from build123d import *

# Parameters (mm, degrees)
EXTRUDE_1_DEPTH     = 2
CUT_EXTRUDE_2_DEPTH = 3


with BuildPart() as part:
    # Эскиз2 → Бобышка-Вытянуть1 (new body)
    with BuildSketch(Plane(origin=(0, 0, 0), x_dir=(1, 0, 0), z_dir=(0, 1, 0))):
        with BuildLine():
            ThreePointArc((-34.560822595, -73.294650793), (-29.912438938, -99.847233064), (-35.042219755, -126.311028042))
            ThreePointArc((-35.042219755, -126.311028042), (-8.723554926, -145.4763519), (4.999999999, -175))
            ThreePointArc((4.999999999, -175), (18.723554924, -145.4763519), (45.042219753, -126.311028042))
            ThreePointArc((45.042219753, -126.311028042), (39.912438936, -99.847233064), (44.560822593, -73.294650793))
            ThreePointArc((44.560822593, -73.294650793), (19.227048475, -55.497690672), (4.999999999, -28))
            ThreePointArc((4.999999999, -28), (-9.227048477, -55.497690672), (-34.560822595, -73.294650793))
        make_face()
    extrude(amount=EXTRUDE_1_DEPTH)

    # Эскиз5 → Вырез-Вытянуть2 (cut, through all)
    with BuildSketch(Plane(origin=(0, 2, 0), x_dir=(1, 0, 0), z_dir=(0, 1, 0))):
        with BuildLine():
            ThreePointArc((1.1922114, -102.391848867), (9.263771174, -100.007354542), (1.1922114, -97.622860217))
            ThreePointArc((1.1922114, -97.622860217), (3.802790428, -100.007354542), (1.1922114, -102.391848867))
        make_face()
        with BuildLine():
            ThreePointArc((-1.894766012, -94.327614743), (4.875778497, -91.169950109), (11.646323005, -94.327614743))
            add(Edge.make_bspline(
                [(11.646323005, -94.327614743), (10.113303771, -87.718633088), (4.875778497, -83.368495621)],
                knots=[0, 0, 0, 1, 1, 1], degree=2))
            add(Edge.make_bspline(
                [(-1.894766012, -94.327614743), (-0.361746778, -87.718633088), (4.875778497, -83.368495621)],
                knots=[0, 0, 0, 1, 1, 1], degree=2))
        make_face()
        with BuildLine():
            add(Edge.make_bspline(
                [(11.646323005, -105.687094341), (10.113303771, -112.296075996), (4.875778497, -116.646213463)],
                knots=[0, 0, 0, 1, 1, 1], degree=2))
            ThreePointArc((11.646323005, -105.687094341), (4.875778497, -108.844758976), (-1.894766012, -105.687094341))
            add(Edge.make_bspline(
                [(-1.894766012, -105.687094341), (-0.361746778, -112.296075996), (4.875778497, -116.646213463)],
                knots=[0, 0, 0, 1, 1, 1], degree=2))
        make_face()
        with BuildLine():
            ThreePointArc((6.916781621, -81.95103194), (14.912317424, -99.810070996), (7.206797889, -117.796144427))
            add(Edge.make_bspline(
                [(6.916781621, -81.95103194), (12.307611516, -78.787526654), (22.389316178, -80.793310488), (29.731357531, -92.811077081), (30.434704422, -105.116682284), (25.64381117, -115.001664232), (17.091486552, -120.227210357), (10.646188457, -120.056173748), (7.206797889, -117.796144427)],
                knots=[0, 0, 0, 0, 0.238043411, 0.386081267, 0.575651621, 0.751375083, 0.825495316, 1, 1, 1, 1], degree=3))
        make_face()
        with BuildLine():
            ThreePointArc((2.544759104, -117.796144427), (-5.160760431, -99.810070996), (2.834775372, -81.95103194))
            add(Edge.make_bspline(
                [(2.834775372, -81.95103194), (-2.556054523, -78.787526654), (-12.637759184, -80.793310488), (-19.979800538, -92.811077081), (-20.683147428, -105.116682284), (-15.892254177, -115.001664232), (-7.339929559, -120.227210357), (-0.894631464, -120.056173748), (2.544759104, -117.796144427)],
                knots=[0, 0, 0, 0, 0.238043411, 0.386081267, 0.575651621, 0.751375083, 0.825495316, 1, 1, 1, 1], degree=3))
        make_face()
    extrude(amount=-CUT_EXTRUDE_2_DEPTH, mode=Mode.SUBTRACT)


solid = part.part
Part model, mm, in its own coordinate system. Coordinates: 2 decimals unless noted, no trailing zeros. Order: outer loops, then holes, each group sorted by start corner. A loop starts at its lowest first (then second) coordinate and runs counter-clockwise, first axis right, second up. Notation, with made-up numbers: M 50.5,76.5 L 84.5,76.5 A12 ccw 84.5,87.5 Z; hole C -2.5,55 d5. An arc over 180 degrees is marked long. One line per question, with ' | ' between items.
Q1. Two-plate mould, pull along X, no slides. Class faces 1 (the face through (9.26, 1.01, 100.17)), 2 (the face through (19.52, 0.99, 55.83)), 3 (the face through (-8.94, 0.986, 55.167)): +X half, -X half, draft (parallel to the pull), parting line (faces both ways), or undercut.
A:
face 1: undercut | face 2: +X half | face 3: -X half
Q2. Drill centre lines: line 1 (X direction, y = 1.9, z = 95); line 2 (Z direction, x = -0.5, y = 1.6); line 3 (X direction, y = 0.4, z = 91). Where is each one in solid material? Low to high.
A:
line 1: x = -30.03 to -19.51, -4.64 to 14.39, 29.26 to 40.03 | line 2: z = 42.7 to 80.56, 85.67 to 90.26, 92.99 to 107.02, 109.76 to 114.35, 119.19 to 158.28 | line 3: x = -30.36 to -18.28, -3.44 to -0.83, 10.58 to 13.19, 28.03 to 40.36
Q3. Slice it at C-C (z = 41). Give the cut face in (x, y).
A:
outline: M 0.35,0 L 9.65,0 L 9.65,2 L 0.35,2 Z
Q4. Slice it at A-A (z = 88). Count the separate pieces of the cut face and the enclosed holes in it, and give its area (3 significant figures).
A:
separate pieces: 4 | enclosed holes: 0 | area: 67.4 mm^2
Q5. Slice it at D-D (z = 160.5). Give the cut face in (x, y).
A:
outline: M 0.53,0 L 9.47,0 L 9.47,2 L 0.53,2 Z
